```python
from build123d import *

# Parameters (mm, degrees)
SKETCH1_W           = 457.2
SKETCH1_H           = 10.16
BOSS_EXTRUDE1_DEPTH = 2.54
SKETCH2_R           = 3.175
BOSS_EXTRUDE2_DEPTH = 1.27
LPATTERN1_COUNT     = 23
LPATTERN1_PITCH     = 19.05


with BuildPart() as part:
    # Sketch1 → Boss-Extrude1 (new body)
    with BuildSketch(Plane.XY):
        with Locations((228.6, 5.08)):
            Rectangle(SKETCH1_W, SKETCH1_H)
    extrude(amount=BOSS_EXTRUDE1_DEPTH)

    # Sketch2 → Boss-Extrude2 (add)
    with BuildSketch(Plane(origin=(0, 0, 0), x_dir=(-1, 0, 0), z_dir=(0, 0, -1))):
        with Locations((-447.675, 4.7625)):
            Circle(SKETCH2_R)
    boss_extrude2 = extrude(amount=BOSS_EXTRUDE2_DEPTH)

    # LPattern1: Boss-Extrude2 ×23
    with Locations(*[(-i * LPATTERN1_PITCH, 0, 0) for i in range(1, LPATTERN1_COUNT)]):
        add(boss_extrude2)


solid = part.part
```
Design review of the part built by this model. Coordinates are the model's own, in mm. Round coordinates to 2 decimals unless told otherwise and drop trailing zeros. Write each loop counter-clockwise with the first axis right and the second up, starting at its lowest first coordinate (ties: lowest second). Pieces come first, ordered by that corner, then holes.
Item 1: The part is to be moulded in two halves that separate along X. For faces 1 (the flat face through (225, 5, 0)), 2 (the flat face through (225, 5, 2.54)), say which applies: +X half, -X half, draft (parallel to the pull), parting line (faces both ways), or undercut.
Item 2: For probe 1 along Z at (x, y) = (432, 8.25); probe 2 along Y at (x, z) = (256.5, -0.45); probe 3 along Y at (x, z) = (411, -0.3), list the stretches that pass through material, from the lowest coordinate up.
Item 3: We need section A-A on x = 287.5. Write out the cut boundary in (y, z), and give its area (3 significant figures).
Returned:
1. face 1: undercut
1. face 2: draft
2. probe 1: z = 0 to 2.54
2. probe 2: y = 1.66 to 7.86
2. probe 3: y = 1.93 to 7.6
3. outline: (0, 0) - (10.16, 0) - (10.16, 2.54) - (0, 2.54) - close
3. area: 25.8 mm2
